from build123d import *

# Parameters (mm, degrees)
BOSS_EXTRUDE1_DEPTH = 5.08
CUT_EXTRUDE1_DEPTH  = 5.08
SKETCH3_R           = 0.762
CUT_EXTRUDE2_DEPTH  = 5.08


with BuildPart() as part:
    # Sketch1 → Boss-Extrude1 (new body)
    with BuildSketch(Plane.XY):
        with BuildLine():
            Line((-8.509, -12.7), (8.509, -12.7))
            ThreePointArc((8.509, -12.7), (11.47248452, -11.47248452), (12.7, -8.509))
            Line((12.7, -8.509), (12.7, 8.509))
            ThreePointArc((12.7, 8.509), (11.47248452, 11.47248452), (8.509, 12.7))
            Line((8.509, 12.7), (-8.509, 12.7))
            ThreePointArc((-8.509, 12.7), (-11.47248452, 11.47248452), (-12.7, 8.509))
            Line((-12.7, 8.509), (-12.7, -8.509))
            ThreePointArc((-12.7, -8.509), (-11.47248452, -11.47248452), (-8.509, -12.7))
        make_face()
    extrude(amount=BOSS_EXTRUDE1_DEPTH)

    # Sketch2 → Cut-Extrude1 (cut)
    with BuildSketch(Plane(origin=(0, 0, 0), x_dir=(-1, 0, 0), z_dir=(0, 0, -1))):
        Polygon((-2.7559, 2.5654), (0, 2.5654), (0, 4.953), (-3.4544, 4.953), (-3.4544, 3.7592), align=None)
        Polygon((0, 4.953), (0, 2.5654), (2.7559, 2.5654), (3.4544, 3.7592), (3.4544, 4.953), align=None)
        with BuildLine():
            ThreePointArc((-7.5692, -2.8956), (-6.34168452, 0.06788452), (-3.3782, 1.2954))
            Line((-3.3782, 1.2954), (3.3782, 1.2954))
            ThreePointArc((3.3782, 1.2954), (6.34168452, 0.06788452), (7.5692, -2.8956))
            Line((7.5692, -2.8956), (7.5692, -5.969))
            ThreePointArc((7.5692, -5.969), (6.34168452, -8.93248452), (3.3782, -10.16))
            Line((3.3782, -10.16), (-3.3782, -10.16))
            ThreePointArc((-3.3782, -10.16), (-6.34168452, -8.93248452), (-7.5692, -5.969))
            Line((-7.5692, -5.969), (-7.5692, -2.8956))
        make_face()
    extrude(amount=-CUT_EXTRUDE1_DEPTH, mode=Mode.SUBTRACT)

    # Sketch3 → Cut-Extrude2 (cut)
    with BuildSketch(Plane(origin=(0, 0, 0), x_dir=(-1, 0, 0), z_dir=(0, 0, -1))):
        with Locations((10.287, -10.287)):
            Circle(SKETCH3_R)
        with Locations((-10.287, -10.287)):
            Circle(SKETCH3_R)
        with Locations((-10.287, 10.287)):
            Circle(SKETCH3_R)
        with Locations(Location((10.287, 10.287, 0), (0, 0, 180))):
            Circle(SKETCH3_R)
    extrude(amount=-CUT_EXTRUDE2_DEPTH, mode=Mode.SUBTRACT)


solid = part.part
Source: CAD feature listing. Evaluate the final solid. Frame: model axes, mm. A direction names the side the tool comes from. Coordinates: 2 decimals unless noted, no trailing zeros. Loops run counter-clockwise (first coordinate to the right, second up) from the corner with the lowest first, then second, coordinate; pieces in that order, holes last. Notation, with made-up numbers: (64.5, -25) - (89.5, -25) arc R14 ccw to (89.5, -18) - close; hole circle Ø5 at (76.5, -30.75). An arc over 180 degrees is marked (long way). Return JSON: item names as keys, results as strings.
Q1. Section B-B, the plane x = 4.5. Return loops of the section in (y, z).
Results:
{"outline": "(-12.7, 0) - (-10.01, 0) - (-10.01, 5.08) - (-12.7, 5.08) - close; (1.14, 0) - (12.7, 0) - (12.7, 5.08) - (1.14, 5.08) - close"}
Q2. Section D-D, the plane z = 4.1. Return loops of the section in (x, y) (3 decimals), plus the area to 3 significant figures.
Results:
{"outline": "(-12.7, -8.509) arc R4.191 ccw to (-8.509, -12.7) - (8.509, -12.7) arc R4.191 ccw to (12.7, -8.509) - (12.7, 8.509) arc R4.191 ccw to (8.509, 12.7) - (-8.509, 12.7) arc R4.191 ccw to (-12.7, 8.509) - close; hole circle Ø1.524 at (-10.287, -10.287); hole circle Ø1.524 at (-10.287, 10.287); hole (-7.569, -5.969) arc R4.191 ccw to (-3.378, -10.16) - (3.378, -10.16) arc R4.191 ccw to (7.569, -5.969) - (7.569, -2.896) arc R4.191 ccw to (3.378, 1.295) - (-3.378, 1.295) arc R4.191 ccw to (-7.569, -2.896) - close; hole (-3.454, 3.759) - (-2.756, 2.565) - (2.756, 2.565) - (3.454, 3.759) - (3.454, 4.953) - (-3.454, 4.953) - close; hole circle Ø1.524 at (10.287, -10.287); hole circle Ø1.524 at (10.287, 10.287)", "area": "449 mm2"}
Q3. Section C-C, the plane x = -10.75. Return loops of the section in (y, z).
Results:
{"outline": "(-12.05, 0) - (-10.89, 0) - (-10.89, 5.08) - (-12.05, 5.08) - close; (-9.68, 0) - (9.68, 0) - (9.68, 5.08) - (-9.68, 5.08) - close; (10.89, 0) - (12.05, 0) - (12.05, 5.08) - (10.89, 5.08) - close"}
Q4. Material intervals for line 1 along Y through (x, z) = (-0.75, 1.25); line 2 along X through (y, z) = (4.5, 1.1); line 3 along Y through (x, z) = (10.75, 4.85), sorted ascending.
Results:
{"line 1": "-12.7 to -10.16, 1.3 to 2.57, 4.95 to 12.7", "line 2": "-12.7 to -3.45, 3.45 to 12.7", "line 3": "-12.05 to -10.89, -9.68 to 9.68, 10.89 to 12.05"}
Q5. Access query for faces 1 (the flat face through (3.454, 4, 3)), 2 (the flat face through (12.7, 0, 3)). Directions: +Z, -Z, +X, -X, +Y, -Y. A direction counts if a zero-diameter tool reaches every point of the face in a straight line with its end or side. Return the directions, or none.
Results:
{"face 1": "+Z, -Z", "face 2": "+Z, -Z, +X, +Y, -Y"}
Q6. Contact query for a flat-ended pin moving along its axis: P1, Ø1.2, axis at x = -10.287, y = -10.287, coming from the +Z side. Output: stop coordinate, or through.
Results:
{"P1": "through"}
Q7. Section A-A, the plane y = -1.5. Return loops of the section in (x, z).
Results:
{"outline": "(-12.7, 0) - (-7.33, 0) - (-7.33, 5.08) - (-12.7, 5.08) - close; (7.33, 0) - (12.7, 0) - (12.7, 5.08) - (7.33, 5.08) - close"}
Q8. Mould query, pull axis X, two halves, no side actions, for faces 3 (the cylindrical face through (-6.374, -8.9, 2.504)), 4 (the flat face through (-12.7, 0, 3)), 5 (the flat face through (0, 6, 0)). Classes: released by +X, released by -X, zero draft, split by the parting line, or undercut.
Results:
{"face 3": "undercut", "face 4": "released by -X", "face 5": "zero draft"}
